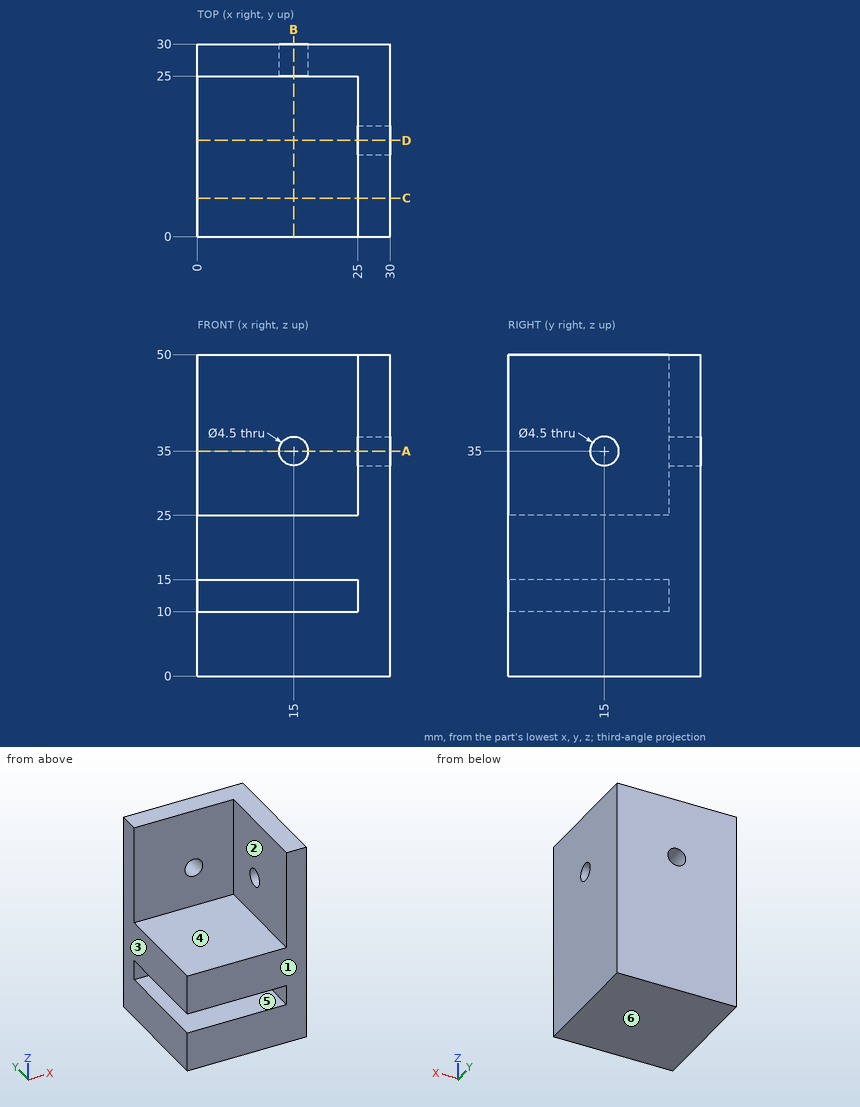
Geometry: see drawing. Coordinates: mm, zero at the bounding-box minimum. A direction names the side the tool comes from. Round coordinates to 2 decimals unless told otherwise and drop trailing zeros. Write each loop counter-clockwise with the first axis right and the second up, starting at its lowest first coordinate (ties: lowest second). Pieces come first, ordered by that corner, then holes. Notation, with made-up numbers: M 8,-9 L 61,-9 A16 cw 61,4 Z; hole C 69.25,-22 d9. An arc over 180 degrees is marked long. Answer as a JSON object with one key per item and string values. Group by question number.
(1) Section query B-B on x = 15. Output: boundary loops of the cut face in (y, z), then the cut area to 4 significant figures.
(2) Mould query, pull axis Z, two halves, no side actions, for the marked faces 3, 4, 5 and 6. Classes: +Z half, -Z half, draft (parallel to the pull), parting line (faces both ways), or undercut.
(3) Reachability of the marked faces 1 and 2 from +Z, -Z, +X, -X, +Y, -Y: full face, straight path, thin tool, end or side. Return the list, or none.
(4) Section query C-C on y = 6. Output: boundary loops of the cut face in (x, z), then the cut area to 3 significant figures.
(5) First-contact query: pin 1 (7.5 mm diameter, centred on x = 8.5, y = 11.5, fed in from +Z); pin 2 (5 mm diameter, centred on x = 15, z = 35, fed in from -Y); pin 3 (5 mm diameter, centred on y = 19.5, z = 35, fed in from -X); pin 4 (2.5 mm diameter, centred on y = 15, z = 35, fed in from -X). Flat tips, straight axial feed; report the tip coordinate or a pass-through.
(6) Section query A-A on z = 35. Output: boundary loops of the cut face in (x, y), then the cut area to 3 significant figures.
(7) Ray query, line 1 (Z direction, x = 7, y = 6); line 2 (Y direction, x = 26.75, z = 35). Return the intervals inside material, ascending. Write a range as [from, to].
Computed values:
{
 "1": {"outline": "M 0,0 L 30,0 L 30,32.75 L 25,32.75 L 25,25 L 0,25 L 0,15 L 25,15 L 25,10 L 0,10 Z; M 25,37.25 L 30,37.25 L 30,50 L 25,50 Z", "area": "727.5 mm^2"},
 "2": {"face 3": "draft", "face 4": "+Z half", "face 5": "undercut", "face 6": "-Z half"},
 "3": {"face 1": "+Z, -Z, +X, -X, -Y", "face 2": "+Z, -X, -Y"},
 "4": {"outline": "M 0,0 L 30,0 L 30,50 L 25,50 L 25,25 L 0,25 L 0,15 L 25,15 L 25,10 L 0,10 Z", "area": "750 mm^2"},
 "5": {"pin 1": "z = 25", "pin 2": "y = 25", "pin 3": "x = 25", "pin 4": "through"},
 "6": {"outline": "M 0,25 L 12.75,25 L 12.75,30 L 0,30 Z; M 17.25,25 L 25,25 L 25,17.25 L 30,17.25 L 30,30 L 17.25,30 Z; M 25,0 L 30,0 L 30,12.75 L 25,12.75 Z", "area": "230 mm^2"},
 "7": {"line 1": "[0, 10], [15, 25]", "line 2": "[0, 12.75], [17.25, 30]"}
}
